Here's how the part is built. I have some questions about the finished solid (model axes, mm). Face numbers are marked on the shaded views. Coordinates: 2 decimals unless noted, no trailing zeros. Loops run counter-clockwise (first coordinate to the right, second up) from the corner with the lowest first, then second, coordinate; pieces in that order, holes last.
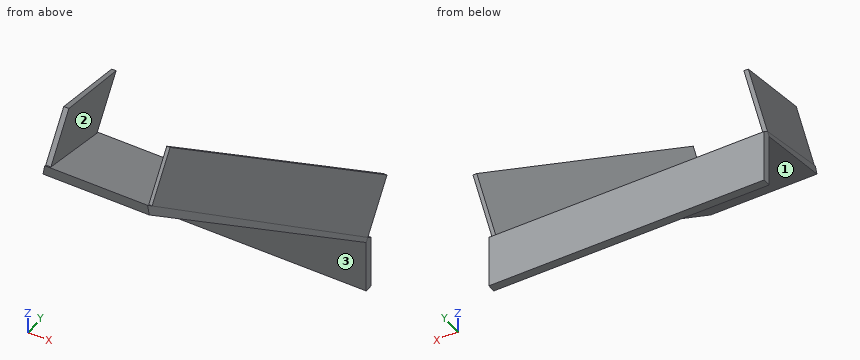
```python
from build123d import *

# Parameters (mm, degrees)
BOSS_EXTRUDE1_DEPTH          = 90
CUT_EXTRUDE_THIN5_DEPTH      = 107.179219538
CUT_EXTRUDE_THIN5_DEPTH_BACK = 90
CUT_EXTRUDE_THIN6_DEPTH      = 107.179219538
CUT_EXTRUDE_THIN6_DEPTH_BACK = 90
BOSS_EXTRUDE2_DEPTH          = 20
BOSS_EXTRUDE3_DEPTH          = 20


with BuildPart() as part:
    # Sketch1 → Boss-Extrude1 (new body)
    with BuildSketch(Plane(origin=(0, 0, 0), x_dir=(0, 0, -1), z_dir=(1, 0, 0))):
        Polygon((-25.714309173, -36.929314965), (25.714309173, 36.929314965), (43.232455695, 36.929314965), (43.232455695, 34.281986352), (25.714309173, 34.281986352), (-22.460611748, -36.929314965), align=None)
    extrude(amount=BOSS_EXTRUDE1_DEPTH)

    # Sketch5 → Cut-Extrude-Thin5 (cut, two sides: drawn at the far end of the back side and taken through both)
    with BuildSketch(Plane(origin=(0, -1.17061758, -1.730385845), x_dir=(-1, 0, 0), z_dir=(0, -0.560329875322556, -0.8282695399572587)).offset(-CUT_EXTRUDE_THIN5_DEPTH_BACK)):
        Polygon((-90, 42.803220717), (-61.682852786, -44.99592237), (-90.234601267, -54.204486788), (-118.551748482, 33.594656299), align=None)
    extrude(amount=CUT_EXTRUDE_THIN5_DEPTH + CUT_EXTRUDE_THIN5_DEPTH_BACK, mode=Mode.SUBTRACT)

    # Sketch6 → Cut-Extrude-Thin6 (cut, two sides: drawn at the far end of the back side and taken through both)
    with BuildSketch(Plane(origin=(0, -1.17061758, -1.730385845), x_dir=(-1, 0, 0), z_dir=(0, -0.560329875322556, -0.8282695399572587)).offset(-CUT_EXTRUDE_THIN6_DEPTH_BACK)):
        Polygon((0, 42.803220717), (-28.102327933, -44.99592237), (0.469772757, -54.141143098), (28.57210069, 33.657999989), align=None)
    extrude(amount=CUT_EXTRUDE_THIN6_DEPTH + CUT_EXTRUDE_THIN6_DEPTH_BACK, mode=Mode.SUBTRACT)

    # Sketch7 → Boss-Extrude2 (add)
    with BuildSketch(Plane(origin=(0, -1.17061758, -1.730385845), x_dir=(-1, 0, 0), z_dir=(0, -0.560329875322556, -0.8282695399572587))):
        Polygon((-88.752727637, 42.803220717), (-61.177479126, -43.172778497), (-62.270856627, -43.172778497), (-90, 42.803220717), align=None)
    extrude(amount=-BOSS_EXTRUDE2_DEPTH)

    # Sketch8 → Boss-Extrude3 (add)
    with BuildSketch(Plane(origin=(0, -1.17061758, -1.730385845), x_dir=(-1, 0, 0), z_dir=(0, -0.560329875322556, -0.8282695399572587))):
        Polygon((0, 42.803220717), (-1.455878042, 42.803220717), (-29.184434589, -43.172778497), (-27.518784801, -43.172778497), align=None)
    extrude(amount=-BOSS_EXTRUDE3_DEPTH)


solid = part.part
```
1. We'd pull the mould along Z, two halves only. Please class the marked faces 1, 2 and 3: +Z half, -Z half, draft (parallel to the pull), parting line (faces both ways), or undercut.
2. I need wall thicknesses on line 1 along Y through (x, z) = (40, -27); line 2 along X through (y, z) = (35, -16); line 3 along X through (y, z) = (13.5, 7.5). Which ranges of each line are inside material? Lowest first, please.
3. I want a section at D-D (y = -3). Please give me the cut outline in (x, z), then the cut area to 3 significant figures.
4. I want a section at B-B (x = 31.5). Please give me the cut outline in (y, z), then the cut area to 3 significant figures.
5. I want a section at A-A (y = 39). Please give me the cut outline in (x, z).
6. For pin 1 (10 mm diameter, centred on y = 35, z = -10.5, fed in from +X); pin 2 (1 mm diameter, centred on x = 32, z = -31.5, fed in from +Y); pin 3 (3 mm diameter, centred on x = 35.5, y = -20.5, fed in from -Z), each with a flat end and sliding along its axis, tell me the tip position at first contact or that it passes through.
7. I want a section at C-C (z = 29). Please give me the cut outline in (x, y).
Response values:
1. face 1: -Z half
1. face 2: undercut
1. face 3: draft
2. line 1: y = 34.28 to 36.93
2. line 2: x = 1.55 to 3.02, 87.2 to 88.44
2. line 3: x = 11.47 to 13.01, 77.26 to 78.45
3. outline: (14.41, -0.49) - (75.48, -0.49) - (71.12, 23.65) - (69.98, 23.65) - (73.85, 2.09) - (16.44, 2.09) - (20.34, 23.65) - (18.74, 23.65) - close
3. area: 216 mm2
4. outline: (-36.93, 22.46) - (34.28, -25.71) - (34.28, -43.23) - (36.93, -43.23) - (36.93, -25.71) - (-36.93, 25.71) - close
4. area: 230 mm2
5. outline: (0, -18.74) - (1.46, -18.74) - (3.98, -4.76) - (2.51, -4.76) - close; (86.24, -4.76) - (88.75, -18.74) - (90, -18.74) - (87.47, -4.76) - close
6. pin 1: stops at x = 89.05
6. pin 2: stops at y = 36.93
6. pin 3: stops at z = 10.33
7. outline: (21.79, -10.9) - (27.52, -32.51) - (29.18, -32.51) - (23.41, -10.9) - close; (61.18, -32.51) - (62.27, -32.51) - (68.04, -10.9) - (66.92, -10.9) - close
